Source: CAD feature listing. Evaluate the final solid. Frame: model axes, mm. Face numbers are marked on the shaded views. A direction names the side the tool comes from. Round coordinates to 2 decimals unless told otherwise and drop trailing zeros. Write each loop counter-clockwise with the first axis right and the second up, starting at its lowest first coordinate (ties: lowest second). Pieces come first, ordered by that corner, then holes. Notation, with made-up numbers: M -38.75,-8 L 6.25,-8 A26 ccw 6.25,22 Z; hole C 68,52.25 d5. An arc over 180 degrees is marked long. Answer in a Markdown table with one row per item.
from build123d import *

# Parameters (mm, degrees)
EXTRUDE_1_DEPTH     = 11.5
SKETCH_2_W          = 5.5
SKETCH_2_H          = 8.4
EXTRUDE_2_DEPTH     = 3.2
SKETCH_3_R          = 1.125
CUT_EXTRUDE_1_DEPTH = 4.2
CUT_EXTRUDE_2_DEPTH = 1.8
FILLET_2_R          = 2
FILLET_3_R          = 1.5


with BuildPart() as part:
    # 草图1 → 凸台-拉伸1 (new body)
    with BuildSketch(Plane.XY):
        Polygon((13.1, 0), (14.4, 0), (14.4, 12), (0, 12), (0, 0), (1.3, 0), (1.3, 9.85), (13.1, 9.85), align=None)
    extrude(amount=EXTRUDE_1_DEPTH)

    # 草图2 → 凸台-拉伸2 (add)
    with BuildSketch(Plane.XZ):
        with Locations((-2.75, 4.2)):
            Rectangle(SKETCH_2_W, SKETCH_2_H)
        with Locations((17.15, 4.2)):
            Rectangle(SKETCH_2_W, SKETCH_2_H)
    extrude(amount=-EXTRUDE_2_DEPTH)

    # 草图3 → 切除-拉伸1 (cut, through all)
    with BuildSketch(Plane(origin=(0, 3.2, 0), x_dir=(1, 0, 0), z_dir=(0, 1, 0))):
        with Locations((-1.6, -4.2)):
            Circle(SKETCH_3_R)
        with Locations((16, -4.2)):
            Circle(SKETCH_3_R)
    extrude(amount=-CUT_EXTRUDE_1_DEPTH, mode=Mode.SUBTRACT)

    # 草图4 → 切除-拉伸2 (cut)
    with BuildSketch(Plane(origin=(0, 3.2, 0), x_dir=(1, 0, 0), z_dir=(0, 1, 0))):
        Polygon((-1.6, -2.352479139), (-3.2, -3.276239569), (-3.2, -5.123760431), (-1.6, -6.047520861), (0, -5.123760431), (0, -3.276239569), align=None)
        Polygon((16, -2.352479139), (14.4, -3.276239569), (14.4, -5.123760431), (16, -6.047520861), (17.6, -5.123760431), (17.6, -3.276239569), align=None)
    extrude(amount=-CUT_EXTRUDE_2_DEPTH, mode=Mode.SUBTRACT)

    # 圆角2
    fillet_2_edges = [part.edges().sort_by_distance(p)[0] for p in [
        (0, 12, 5.75),
        (14.4, 12, 5.75),
    ]]
    fillet(fillet_2_edges, radius=FILLET_2_R)

    # 圆角3
    fillet_3_edges = [part.edges().sort_by_distance(p)[0] for p in [
        (13.1, 9.85, 5.75),
        (1.3, 9.85, 5.75),
    ]]
    fillet(fillet_3_edges, radius=FILLET_3_R)


solid = part.part
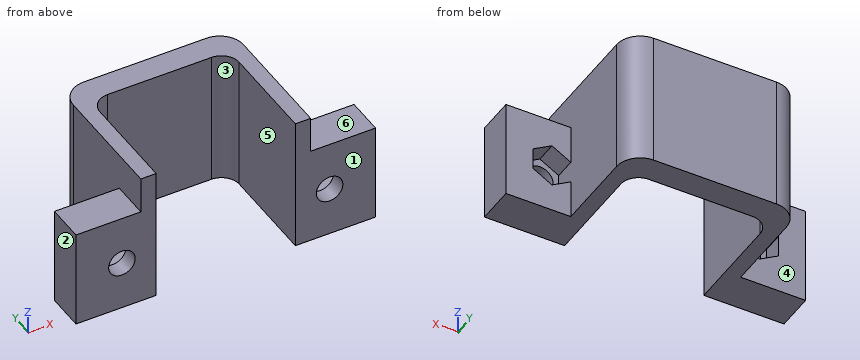
Q1. Section C-C (y = 3.5). Return loops of the section in (x, z).
Solutions:
| item | result |
|---|---|
| outline | M 0,0 L 1.3,0 L 1.3,11.5 L 0,11.5 Z; M 13.1,0 L 14.4,0 L 14.4,11.5 L 13.1,11.5 Z |
Q2. Material intervals for probe 1 along X at (y, z) = (0.5, 4.2) (3 decimals); probe 2 along X at (y, z) = (2.5, 5); probe 3 along Z at (x, y) = (-1.6, 0.7) (3 decimals), sorted ascending.
Solutions:
| item | result |
|---|---|
| probe 1 | x = -5.5 to -2.725, -0.475 to 1.3, 13.1 to 14.875, 17.125 to 19.9 |
| probe 2 | x = -5.5 to -3.2, 0 to 1.3, 13.1 to 14.4, 17.6 to 19.9 |
| probe 3 | z = 0 to 3.075, 5.325 to 8.4 |
Q3. Section A-A (y = 1). Return loops of the section in (x, z) (3 decimals), and give its area (3 significant figures).
Solutions:
| item | result |
|---|---|
| outline | M -5.5,0 L 1.3,0 L 1.3,11.5 L 0,11.5 L 0,8.4 L -5.5,8.4 Z; M 13.1,0 L 19.9,0 L 19.9,8.4 L 14.4,8.4 L 14.4,11.5 L 13.1,11.5 Z; hole C -1.6,4.2 d2.25; hole C 16,4.2 d2.25 |
| area | 114 mm2 |
Q4. Access query for the marked faces 4, 5 and 6. Directions: +Z, -Z, +X, -X, +Y, -Y. A direction counts if a zero-diameter tool reaches every point of the face in a straight line with its end or side. Return the directions, or none.
Solutions:
| item | result |
|---|---|
| face 4 | +Z, -Z, -X, +Y |
| face 5 | +Z, -Z, -Y |
| face 6 | +Z, +X, +Y, -Y |
Q5. Section B-B (z = 4.2). Return loops of the section in (x, y) (3 decimals).
Solutions:
| item | result |
|---|---|
| outline | M -5.5,0 L -2.725,0 L -2.725,1.4 L -3.2,1.4 L -3.2,3.2 L -5.5,3.2 Z; M -0.475,0 L 1.3,0 L 1.3,8.35 A1.5 cw 2.8,9.85 L 11.6,9.85 A1.5 cw 13.1,8.35 L 13.1,0 L 14.875,0 L 14.875,1.4 L 14.4,1.4 L 14.4,10 A2 ccw 12.4,12 L 2,12 A2 ccw 0,10 L 0,1.4 L -0.475,1.4 Z; M 17.125,0 L 19.9,0 L 19.9,3.2 L 17.6,3.2 L 17.6,1.4 L 17.125,1.4 Z |
Q6. Section D-D (z = 1). Return loops of the section in (x, y), and give its area (3 significant figures).
Solutions:
| item | result |
|---|---|
| outline | M -5.5,0 L 1.3,0 L 1.3,8.35 A1.5 cw 2.8,9.85 L 11.6,9.85 A1.5 cw 13.1,8.35 L 13.1,0 L 19.9,0 L 19.9,3.2 L 14.4,3.2 L 14.4,10 A2 ccw 12.4,12 L 2,12 A2 ccw 0,10 L 0,3.2 L -5.5,3.2 Z |
| area | 91.0 mm2 |
Q7. Pull-direction query (X, two-part tool) for the marked faces 1, 2 and 3; classes: pulls with the +X half, pulls with the -X half, needs draft (parallel to the pull), parting line crosses it, or undercut.
Solutions:
| item | result |
|---|---|
| face 1 | needs draft |
| face 2 | pulls with the -X half |
| face 3 | undercut |
Q8. Contact query for flat-ended pins moving along their axis: pin 1 Ø1.6 at (x, z) = (18, 2.5) entering from +Y; pin 2 Ø1.6 at (x, z) = (-1.5, 3.5) entering from +Y; pin 3 Ø1 at (x, y) = (-2.5, 1) entering from +Z; pin 4 Ø1.3 at (x, z) = (-1.6, 4.2) entering from +Y. Output: stop coordinate, or through.
Solutions:
| item | result |
|---|---|
| pin 1 | stops at y = 3.2 |
| pin 2 | stops at y = 1.4 |
| pin 3 | stops at z = 8.4 |
| pin 4 | passes through |
